```python
from build123d import *

# Parameters (mm, degrees)
F0_W     = 5.5
F0_H     = 14.3
F1_DEPTH = 5.2
F2_W     = 2
F2_H     = 12.5
F3_DEPTH = 5.5
F5_W     = 5.5
F5_H     = 1.5
F6_DEPTH = 2.15
F7_R     = 1.25
F8_DEPTH = 3


with BuildPart() as f1:
    # F0 (on Front) → F1 (new body)
    with BuildSketch(Plane.XZ):
        with Locations((0, 7.15)):
            Rectangle(F0_W, F0_H)
    extrude(amount=F1_DEPTH)

    # F2 (on face) → F3 (cut)
    with BuildSketch(Plane.XZ.offset(5.2)):
        with Locations((0, 6.25)):
            Rectangle(F2_W, F2_H)
        with BuildLine():
            ThreePointArc((1, 12.5), (0, 13.5), (-1, 12.5))
            Line((-1, 12.5), (1, 12.5))
        make_face()
    extrude(amount=-F3_DEPTH, mode=Mode.SUBTRACT)

    # F5 (on offset) → F6 (join)
    with BuildSketch(Plane.XZ.offset(1.55)):
        with Locations((0, 15.05)):
            Rectangle(F5_W, F5_H)
        with BuildLine():
            ThreePointArc((2.75, 15.8), (0, 18.55), (-2.75, 15.8))
            Line((-2.75, 15.8), (2.75, 15.8))
        make_face()
    extrude(amount=F6_DEPTH)

    # F7 (on face) → F8 (cut)
    with BuildSketch(Plane.XZ.offset(3.7)):
        with Locations((0, 17)):
            Circle(F7_R)
    extrude(amount=-F8_DEPTH, mode=Mode.SUBTRACT)

    # F9: F1 across plane


with BuildPart() as f1_1:
    add(f1.part)
    add(f1.part.mirror(Plane.XY))


solid = f1_1.part
```
Design review of the part built by this model. Coordinates are the model's own, in mm. A direction names the side the tool comes from. Coordinates: 2 decimals unless noted, no trailing zeros. Loops run counter-clockwise (first coordinate to the right, second up) from the corner with the lowest first, then second, coordinate; pieces in that order, holes last. Notation, with made-up numbers: (-25, -24.5) - (-15, -24.5) arc R19 ccw to (-15, 6.5) - close; hole circle Ø6 at (-28.75, 86). An arc over 180 degrees is marked (long way). Use CSV: the item, a comma, the result in double quotes. Start each with the question number.
1) Consider section A-A on z = -11. Write out the cut boundary in (x, y).
2) Consider section C-C on x = 2.3. Write out the cut boundary in (y, z).
3) Tool access review of faces 5 (the flat face through (0, -3.7, -15.5)), 6 (the flat face through (0, -1.55, -15.5)), 7 (the flat face through (0, -4, 14.3)): name each direction out of +Z, -Z, +X, -X, +Y, -Y from which nothing blocks a thin tool from reaching the whole face with its end or side.
4) Consider section B-B on y = -3.3. Write out the cut boundary in (x, z), then the cut area to 3 significant figures.
5) For pin 1 Ø3 at (x, z) = (0, 17) entering from +Y; pin 2 Ø3 at (x, z) = (0, -17) entering from -Y; pin 3 Ø0.5 at (x, y) = (1, -0.5) entering from +Z, all flat-tipped, find the tip position at first contact; note any pin that passes through.
6) Consider section D-D on z = 17. Write out the cut boundary in (x, y), then the cut area to 3 significant figures.
7) Wall thickness on L1, parallel to Z at x = 0, y = -2.55; L2, parallel to X at y = -1.7, z = 9.5; L3, parallel to Z at x = 1.7, y = -1.15: over which ranges is each line inside the solid? List them lowest first. Write a range as from..to.
8) The part is to be moulded in two halves that separate along Z. For faces 1 (the cylindrical face through (0, -2.6, 13.5)), 2 (the flat face through (0, -1.55, 15.5)), 3 (the flat face through (0, -1, -14.3)), 4 (the cylindrical face through (0, -2.6, -13.5)), say which applies: +Z half, -Z half, draft (parallel to the pull), parting line (faces both ways), or undercut.
Geometry says:
1,outline,"(-2.75, -5.2) - (-1, -5.2) - (-1, 0) - (-2.75, 0) - close; (1, -5.2) - (2.75, -5.2) - (2.75, 0) - (1, 0) - close"
2,outline,"(-5.2, -14.3) - (-3.7, -14.3) - (-3.7, -17.31) - (-1.55, -17.31) - (-1.55, -14.3) - (0, -14.3) - (0, 14.3) - (-1.55, 14.3) - (-1.55, 17.31) - (-3.7, 17.31) - (-3.7, 14.3) - (-5.2, 14.3) - close"
3,face 5,"-Z, +X, -X, -Y"
3,face 6,"-Z, +X, -X, +Y"
3,face 7,"+Z, +X, -X, -Y"
4,outline,"(-2.75, -15.8) arc R2.75 ccw to (2.75, -15.8) - (2.75, 15.8) arc R2.75 ccw to (-2.75, 15.8) - close; hole circle Ø2.5 at (0, -17); hole circle Ø2.5 at (0, 17); hole (-1, -12.5) arc R1 ccw to (1, -12.5) - (1, 12.5) arc R1 ccw to (-1, 12.5) - close"
4,area,"135 mm^2"
5,pin 1,"y = -1.55"
5,pin 2,"y = -3.7"
5,pin 3,"z = 14.3"
6,outline,"(-2.47, -3.7) - (-1.25, -3.7) - (-1.25, -1.55) - (-2.47, -1.55) - close; (1.25, -3.7) - (2.47, -3.7) - (2.47, -1.55) - (1.25, -1.55) - close"
6,area,"5.26 mm^2"
7,L1,"-18.55..-18.25, -15.75..-13.5, 13.5..15.75, 18.25..18.55"
7,L2,"-2.75..-1, 1..2.75"
7,L3,"-14.3..14.3"
8,face 1,"undercut"
8,face 2,"draft"
8,face 3,"-Z half"
8,face 4,"undercut"
